```python
from build123d import *

# Parameters (mm, degrees)
SKETCH1_W               = 24
SKETCH1_H               = 141
BOSS_EXTRUDE1_DEPTH     = 1.5
SKETCH2_W               = 3
SKETCH2_H               = 35
CUT_EXTRUDE1_DEPTH      = 2.5
CUT_EXTRUDE1_DEPTH_BACK = 2.5
FILLET1_R               = 3
SKETCH3_W               = 6
SKETCH3_H               = 3
CUT_EXTRUDE2_DEPTH      = 2.5
CUT_EXTRUDE2_DEPTH_BACK = 2.5


with BuildPart() as part:
    # Sketch1 → Boss-Extrude1 (new body, symmetric)
    with BuildSketch(Plane(origin=(0, 0, 0), x_dir=(1, 0, 0), z_dir=(0, 1, 0))):
        Rectangle(SKETCH1_W, SKETCH1_H)
    extrude(amount=BOSS_EXTRUDE1_DEPTH, both=True)

    # Sketch2 → Cut-Extrude1 (cut, two sides)
    with BuildSketch(Plane(origin=(0, 0, 0), x_dir=(1, 0, 0), z_dir=(0, 1, 0))) as cut_extrude1_sk:
        with Locations((-7.5, 28)):
            Rectangle(SKETCH2_W, SKETCH2_H)
        with Locations((7.5, 28)):
            Rectangle(SKETCH2_W, SKETCH2_H)
        with Locations((7.5, -28)):
            Rectangle(SKETCH2_W, SKETCH2_H)
        with Locations((-7.5, -28)):
            Rectangle(SKETCH2_W, SKETCH2_H)
    extrude(amount=CUT_EXTRUDE1_DEPTH, mode=Mode.SUBTRACT)
    extrude(cut_extrude1_sk.sketch, amount=-CUT_EXTRUDE1_DEPTH_BACK, mode=Mode.SUBTRACT)

    # Fillet1
    fillet1_edges = [part.edges().sort_by_distance(p)[0] for p in [
        (-12, 0, -70.5),
        (12, 0, -70.5),
        (12, 0, 70.5),
        (-12, 0, 70.5),
    ]]
    fillet(fillet1_edges, radius=FILLET1_R)

    # Sketch3 → Cut-Extrude2 (cut, two sides)
    with BuildSketch(Plane(origin=(0, 0, 0), x_dir=(1, 0, 0), z_dir=(0, 1, 0))) as cut_extrude2_sk:
        with Locations((0, 69)):
            Rectangle(SKETCH3_W, SKETCH3_H)
    extrude(amount=CUT_EXTRUDE2_DEPTH, mode=Mode.SUBTRACT)
    extrude(cut_extrude2_sk.sketch, amount=-CUT_EXTRUDE2_DEPTH_BACK, mode=Mode.SUBTRACT)


solid = part.part
```
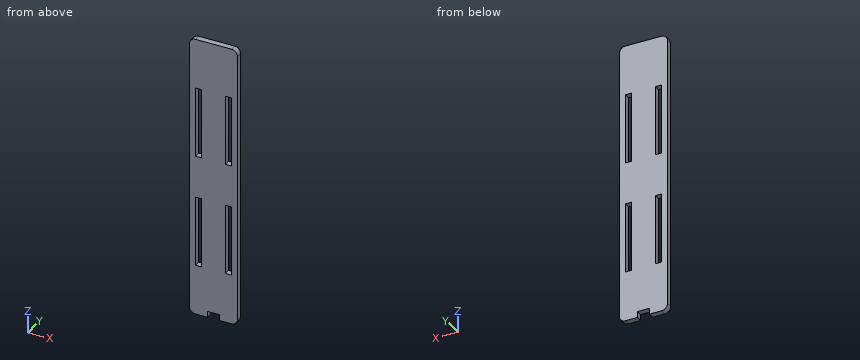
Check sheet for the modelled part. Datum: model origin and axes. Units: mm. Give positions to 0.01 mm unless a question says otherwise; leave off trailing zeros. Write each loop counter-clockwise with the first axis right and the second up, starting at its lowest first coordinate (ties: lowest second). Pieces come first, ordered by that corner, then holes. Notation, with made-up numbers: (35, 35) -> (47, 35) arc R13 ccw to (47, 45) -> close; hole circle Ø8 at (-20.5, 80). An arc over 180 degrees is marked (long way). Use CSV: the item, a comma, the result in double quotes. Start each with the question number.
Q1. Scan lines: line 1 along X through (y, z) = (-0.6, 34.5); line 2 along Z through (x, y) = (-7.25, 0.75); line 3 along Z through (x, y) = (-1.75, 0.3). Record each from-to range of solid material in increasing order.
Q2. Cross-section at C-C on x = 0. Enter the section's corners in (y, z), and give its area (3 significant figures).
Q3. Depth check by flat-ended pin: P1, Ø1.5, axis at y = 0, z = -69.5, coming from the -X side; P2, Ø1, axis at x = -2, y = 0.5, coming from the -Z side. Enter the tip coordinate at first touch or a pass-through.
Q4. Cross-section at A-A on z = 43.5. Enter the section's corners in (x, y).
Q5. Cross-section at B-B on y = 0.45. Enter the section's corners in (x, z), and give its area (3 significant figures).
Working result:
1,line 1,"x = -12 to -9, -6 to 6, 9 to 12"
1,line 2,"z = -70.5 to -45.5, -10.5 to 10.5, 45.5 to 70.5"
1,line 3,"z = -67.5 to 70.5"
2,outline,"(-1.5, -67.5) -> (1.5, -67.5) -> (1.5, 70.5) -> (-1.5, 70.5) -> close"
2,area,"414 mm^2"
3,P1,"stops at x = -11.73"
3,P2,"stops at z = -67.5"
4,outline,"(-12, -1.5) -> (-9, -1.5) -> (-9, 1.5) -> (-12, 1.5) -> close; (-6, -1.5) -> (6, -1.5) -> (6, 1.5) -> (-6, 1.5) -> close; (9, -1.5) -> (12, -1.5) -> (12, 1.5) -> (9, 1.5) -> close"
5,outline,"(-12, -67.5) arc R3 ccw to (-9, -70.5) -> (-3, -70.5) -> (-3, -67.5) -> (3, -67.5) -> (3, -70.5) -> (9, -70.5) arc R3 ccw to (12, -67.5) -> (12, 67.5) arc R3 ccw to (9, 70.5) -> (-9, 70.5) arc R3 ccw to (-12, 67.5) -> close; hole (-9, -45.5) -> (-6, -45.5) -> (-6, -10.5) -> (-9, -10.5) -> close; hole (-9, 10.5) -> (-6, 10.5) -> (-6, 45.5) -> (-9, 45.5) -> close; hole (6, -45.5) -> (9, -45.5) -> (9, -10.5) -> (6, -10.5) -> close; hole (6, 10.5) -> (9, 10.5) -> (9, 45.5) -> (6, 45.5) -> close"
5,area,"2,940 mm^2"
